from build123d import *

# Parameters (mm, degrees)
F0_W     = 50.8
F0_H     = 50.8
F1_DEPTH = 6.35
F2_R     = 5.08
F3_R     = 12.7
F4_DEPTH = 3.175


with BuildPart() as f1:
    # F0 (on Top) → F1 (new body)
    with BuildSketch(Plane.XY):
        Rectangle(F0_W, F0_H)
    extrude(amount=F1_DEPTH)

    # F2
    f2_edges = [f1.edges().sort_by_distance(p)[0] for p in [
        (-25.4, -25.4, 3.175),
        (25.4, -25.4, 3.175),
    ]]
    fillet(f2_edges, radius=F2_R)

    # F3 (on face) → F4 (cut)
    with BuildSketch(Plane.XY.offset(6.35)):
        Circle(F3_R)
    extrude(amount=-F4_DEPTH, mode=Mode.SUBTRACT)


solid = f1.part
Check sheet for the modelled part. Datum: model origin and axes. Units: mm. A direction names the side the tool comes from. Give positions to 0.01 mm unless a question says otherwise; leave off trailing zeros. Write each loop counter-clockwise with the first axis right and the second up, starting at its lowest first coordinate (ties: lowest second). Pieces come first, ordered by that corner, then holes. Notation, with made-up numbers: (-27.5, 20.25) -> (21.5, 20.25) arc R24 ccw to (21.5, 49.25) -> close; hole circle Ø10 at (81, 61.25). An arc over 180 degrees is marked (long way). Write item = value, one per line.
Item 1: Sectioned sample at A-A on z = 5.25. Record the boundary of the cut face in (x, y), and give its area (3 significant figures).
Output:
outline = (-25.4, -20.32) arc R5.08 ccw to (-20.32, -25.4) -> (20.32, -25.4) arc R5.08 ccw to (25.4, -20.32) -> (25.4, 25.4) -> (-25.4, 25.4) -> close; hole circle Ø25.4 at (0, 0)
area = 2,060 mm^2
Item 2: Sectioned sample at B-B on y = 0. Record the boundary of the cut face in (x, z) (3 decimals).
Output:
outline = (-25.4, 0) -> (25.4, 0) -> (25.4, 6.35) -> (12.7, 6.35) -> (12.7, 3.175) -> (-12.7, 3.175) -> (-12.7, 6.35) -> (-25.4, 6.35) -> close
Item 3: Release check for a two-part mould opening along X. For faces 3 (the flat face through (25.4, 2, 3)), 4 (the flat face through (0, 0, 3.175)), 5 (the flat face through (0, 0, 0)) record: +X half, -X half, draft (parallel to the pull), parting line (faces both ways), or undercut.
Output:
face_3 = +X half
face_4 = undercut
face_5 = draft
Item 4: Tool access check on faces 1 (the cylindrical face through (-2.75, -12.4, 4.78)), 2 (the flat face through (-6, 12, 6.35)). Record the directions out of +Z, -Z, +X, -X, +Y, -Y that give a thin tool (end or side, any length) a straight path to the whole face; none if there is none.
Output:
face_1 = +Z
face_2 = +Z, +X, -X, +Y, -Y
Item 5: Scan lines: probe 1 along Y at (x, z) = (0, 5.55); probe 2 along X at (y, z) = (-7.5, 4.5); probe 3 along Z at (x, y) = (8, 2) (3 decimals). Record each from-to range of solid material in increasing order. Write a range as from..to.
Output:
probe_1 = -25.4..-12.7, 12.7..25.4
probe_2 = -25.4..-10.25, 10.25..25.4
probe_3 = 0..3.175
Item 6: Gauge pin test, flat end, axial feed: pin 1 (12 mm diameter, centred on x = -5.5, y = -20, fed in from -Z). Record the tip position at first contact, or that the pin passes through.
Output:
pin_1 = 0
